```python
from build123d import *

# Parameters (mm, degrees)
ESQUISSE1_W                  = 21
ESQUISSE1_H                  = 20
BOSS_EXTRU_1_DEPTH           = 2
ESQUISSE2_W                  = 2
ESQUISSE2_H                  = 20
BOSS_EXTRU_2_DEPTH           = 19
ESQUISSE3_R                  = 2.05
ENL_V_MAT_EXTRU_1_DEPTH      = 20
ESQUISSE4_R                  = 2.05
ENL_V_MAT_EXTRU_2_DEPTH      = 20
ESQUISSE5_W                  = 15
ESQUISSE5_H                  = 1.39480656
BOSS_EXTRU_3_DEPTH           = 15
CHANFREIN1_SIZE              = 15
CONG_1_R                     = 1
BOSS_EXTRU_12_DEPTH          = 4
ENL_V_MAT_EXTRU_3_DEPTH      = 26.51960031
ENL_V_MAT_EXTRU_3_DEPTH_BACK = 26.51960031
ESQUISSE9_R                  = 6.5


with BuildPart() as part:
    # Esquisse1 → Boss.-Extru.1 (new body)
    with BuildSketch(Plane(origin=(0, 0, 0), x_dir=(1, 0, 0), z_dir=(0, 1, 0))):
        Rectangle(ESQUISSE1_W, ESQUISSE1_H)
    extrude(amount=BOSS_EXTRU_1_DEPTH)

    # Esquisse2 → Boss.-Extru.2 (add)
    with BuildSketch(Plane(origin=(0, 2, 0), x_dir=(1, 0, 0), z_dir=(0, 1, 0))):
        with Locations((-9.5, 0)):
            Rectangle(ESQUISSE2_W, ESQUISSE2_H)
    extrude(amount=BOSS_EXTRU_2_DEPTH)

    # Esquisse3 → Enlèv. mat.-Extru.1 (cut)
    with BuildSketch(Plane(origin=(0, 2, 0), x_dir=(1, 0, 0), z_dir=(0, 1, 0))):
        with Locations(Location((-0.5, 0, 0), (0, 0, 270))):
            Circle(ESQUISSE3_R)
    extrude(amount=-ENL_V_MAT_EXTRU_1_DEPTH, mode=Mode.SUBTRACT)

    # Esquisse4 → Enlèv. mat.-Extru.2 (cut)
    with BuildSketch(Plane(origin=(-8.5, 0, 0), x_dir=(0, 0, -1), z_dir=(1, 0, 0))):
        with Locations((0, 11)):
            Circle(ESQUISSE4_R)
    extrude(amount=-ENL_V_MAT_EXTRU_2_DEPTH, mode=Mode.SUBTRACT)

    # Esquisse5 → Boss.-Extru.3 (add)
    with BuildSketch(Plane(origin=(0, 2, 0), x_dir=(1, 0, 0), z_dir=(0, 1, 0))):
        with Locations((-1, -5.69740328)):
            Rectangle(ESQUISSE5_W, ESQUISSE5_H)
        with Locations((-1, 5.69740328)):
            Rectangle(ESQUISSE5_W, ESQUISSE5_H)
    extrude(amount=BOSS_EXTRU_3_DEPTH)

    # Chanfrein1
    chanfrein1_edges = [part.edges().sort_by_distance(p)[0] for p in [
        (6.5, 17, 5.69740328),
        (6.5, 17, -5.69740328),
    ]]
    chamfer(chanfrein1_edges, length=CHANFREIN1_SIZE - 0.0001)  # a hair under: the kernel refuses the full size

    # Congé1
    cong_1_edges = [part.edges().sort_by_distance(p)[0] for p in [
        (10.5, 2, 0),
        (1, 2, 10),
        (-8.5, 21, 0),
        (-8.5, 11.5, 10),
        (-8.5, 11.5, -10),
        (1, 2, -10),
    ]]
    fillet(cong_1_edges, radius=CONG_1_R)

    # Esquisse7 → Boss.-Extru.12 (add)
    with BuildSketch(Plane(origin=(-8.5, 0, 0), x_dir=(0, 0, -1), z_dir=(1, 0, 0))):
        with BuildLine():
            Line((5, 8.708712153), (5, 13.291287847))
            ThreePointArc((5, 13.291287847), (0, 16.5), (-5, 13.291287847))
            Line((-5, 13.291287847), (-5, 8.708712153))
            ThreePointArc((-5, 8.708712153), (0, 5.5), (5, 8.708712153))
        make_face()
        Polygon((3.55, 8.950406544), (0, 6.900813089), (-3.55, 8.950406544), (-3.55, 13.049593456), (0, 15.099186911), (3.55, 13.049593456), align=None, mode=Mode.SUBTRACT)
    extrude(amount=BOSS_EXTRU_12_DEPTH)

    # Esquisse9 → Enlèv. mat.-Extru.3 (cut, two sides: drawn at the far end of the back side and taken through both)
    with BuildSketch(Plane(origin=(0, 0, 0), x_dir=(0, 0, -1), z_dir=(1, 0, 0)).offset(-ENL_V_MAT_EXTRU_3_DEPTH_BACK)):
        with Locations((-10, 21)):
            Circle(ESQUISSE9_R)
        with Locations((10, 21)):
            Circle(ESQUISSE9_R)
    extrude(amount=ENL_V_MAT_EXTRU_3_DEPTH + ENL_V_MAT_EXTRU_3_DEPTH_BACK, mode=Mode.SUBTRACT)


solid = part.part
```
Can you work these out from the model? Positions are in its coordinate system, mm. A direction names the side the tool comes from. Coordinates: 2 decimals unless noted, no trailing zeros. Loops run counter-clockwise (first coordinate to the right, second up) from the corner with the lowest first, then second, coordinate; pieces in that order, holes last. Notation, with made-up numbers: (52, 28.5) -> (70, 28.5) arc R17 cw to (70, 44.5) -> close; hole circle Ø6 at (82, 32.5). An arc over 180 degrees is marked (long way). Put each result on its own line as item: value. Start each with the question number.
Q1. I'm going to push flat-ended pins straight in: P1, Ø5.5, axis at x = 0, z = 1, coming from the +Y side; P2, Ø8, axis at y = 10.5, z = 0, coming from the +X side; P3, Ø1, axis at x = -6, z = -6, coming from the +Y side. Where does each tip first touch, or does it pass through?
Q2. I want a section at C-C (z = -4.25). Write out the boundary of the cut face in (x, y), plus the area to 3 significant figures.
Q3. I want a section at A-A (x = -0.5). Write out the boundary of the cut face in (y, z).
Q4. Thinking about a two-plate mould opening in Y: for faces 6 (the face through (-6.53, 7.91, 1.75)), 7 (the face through (-9.577, 16.354, 5.455)), 8 (the face through (-8.5, 5, 0)), 9 (the face through (1.533, 1.014, -0.267)), which applies, pulls with the +Y half, pulls with the -Y half, needs draft (parallel to the pull), parting line crosses it, or undercut?
Q5. If I drill on line 1 (X direction, y = 0.6, z = 0); line 2 (Z direction, x = 1.5, y = 6.75); line 3 (X direction, y = 6.5, z = -7.5), over which ranges is the centre line in solid material (lowest first)? Write a range as [from, to].
Q6. For faces 1 (the face through (-8.5, 9, 8)), 2 (the face through (-3, 6, 5)), 3 (the face through (-8.5, 17, 0)), 4 (the face through (-3.2, 0.8, 10)), 5 (the face through (-9.486, 8.999, 0.444)), which set-ups out of +Z, -Z, +X, -X, +Y, -Y let a thin tool reach every point of the face, with its end or its side?
Q7. I want a section at B-B (y = 11). Write out the boundary of the cut face in (x, z), plus the area to 3 significant figures.
Q8. I want a section at D-D (z = 2.5). Write out the boundary of the cut face in (x, y), plus the area to 3 significant figures.
Taken from the geometry:
1. P1: stops at y = 2
1. P2: stops at x = -4.5
1. P3: stops at y = 15
2. outline: (-10.5, 0) -> (10.5, 0) -> (10.5, 1) arc R1 ccw to (9.5, 2) -> (-8.5, 2) -> (-8.5, 7.51) -> (-4.5, 7.51) -> (-4.5, 14.49) -> (-8.5, 14.49) -> (-8.5, 17.97) -> (-10.5, 17.97) -> close
2. area: 102 mm2
3. outline: (0, -10) -> (1, -10) arc R1 ccw to (2, -9) -> (2, -6.39) -> (9, -6.39) -> (9, -5) -> (2, -5) -> (2, -2.05) -> (0, -2.05) -> close; (0, 2.05) -> (2, 2.05) -> (2, 5) -> (9, 5) -> (9, 6.39) -> (2, 6.39) -> (2, 9) arc R1 ccw to (1, 10) -> (0, 10) -> close
4. face 6: undercut
4. face 7: pulls with the +Y half
4. face 8: undercut
4. face 9: needs draft
5. line 1: x = [-10.5, -2.55], [1.55, 10.5]
5. line 2: z = [-6.39, -5], [5, 6.39]
5. line 3: x = [-10.5, -8.5]
6. face 1: +Z, +X, +Y
6. face 2: +X
6. face 3: +X, +Y
6. face 4: +Z, +X, -X, +Y, -Y
6. face 5: +X, -X
7. outline: (-10.5, -10) -> (-9.5, -10) arc R1 ccw to (-8.5, -9) -> (-8.5, -6.39) -> (-2.5, -6.39) -> (-2.5, -5) -> (-4.5, -5) -> (-4.5, -3.55) -> (-8.5, -3.55) -> (-8.5, -2.05) -> (-10.5, -2.05) -> close; (-10.5, 2.05) -> (-8.5, 2.05) -> (-8.5, 3.55) -> (-4.5, 3.55) -> (-4.5, 5) -> (-2.5, 5) -> (-2.5, 6.39) -> (-8.5, 6.39) -> (-8.5, 9) arc R1 ccw to (-9.5, 10) -> (-10.5, 10) -> close
7. area: 59.7 mm2
8. outline: (-10.5, 0) -> (10.5, 0) -> (10.5, 1) arc R1 ccw to (9.5, 2) -> (-8.5, 2) -> (-8.5, 6.1) -> (-4.5, 6.1) -> (-4.5, 8.34) -> (-8.5, 8.34) -> (-8.5, 13.66) -> (-4.5, 13.66) -> (-4.5, 15.9) -> (-8.5, 15.9) -> (-8.5, 20) arc R1 ccw to (-9.5, 21) -> (-10.5, 21) -> close
8. area: 97.5 mm2
